from build123d import *

# Parameters (mm, degrees)
SKETCH3_W          = 8.5
SKETCH3_H          = 1
CUT_EXTRUDE1_DEPTH = 12.4
CUT_EXTRUDE2_DEPTH = 12.4


with BuildPart() as part:
    # Sketch1 → Revolve1 (revolve)
    with BuildSketch(Plane(origin=(0, 0, 0), x_dir=(0, 0, -1), z_dir=(1, 0, 0)), mode=Mode.PRIVATE) as revolve1_sk:
        with BuildLine():
            Line((-12.4, 7), (-12.4, 3.675))
            Line((-12.4, 3.675), (-11.9, 3.175))
            Line((-11.9, 3.175), (-0.5, 3.175))
            Line((-0.5, 3.175), (0, 3.675))
            Line((0, 3.675), (0, 8))
            Line((0, 8), (-0.5, 8.5))
            Line((-0.5, 8.5), (-2.2, 8.5))
            Line((-2.2, 8.5), (-2.2, 8.3))
            Line((-2.2, 8.3), (-4.4, 8.3))
            Line((-4.4, 8.3), (-4.4, 8.5))
            Line((-4.4, 8.5), (-7, 8.5))
            Line((-7, 8.5), (-7, 8.1))
            ThreePointArc((-7, 8.1), (-7.175735931, 7.675735931), (-7.6, 7.5))
            Line((-7.6, 7.5), (-11.9, 7.5))
            Line((-11.9, 7.5), (-12.4, 7))
        make_face()
    revolve(revolve1_sk.sketch.rotate(Axis((0, 0, 0), (0, 0, 1)), 270), axis=Axis((0, 0, 0), (0, 0, 1)))

    # Sketch2 → Cut-Revolve1 (revolve, cut)
    with BuildSketch(Plane.XY.offset(3), mode=Mode.PRIVATE) as cut_revolve1_sk:
        Polygon((-6, 8.5), (-3.5, 8.5), (-3.5, 2.3), (-4.9935, 2.3), (-4.9935, -8.5), (-6, -8.5), align=None)
    revolve(cut_revolve1_sk.sketch.rotate(Axis((-6, -8.5, 3), (0, 1, 0)), 270), axis=Axis((-6, -8.5, 3), (0, 1, 0)), mode=Mode.SUBTRACT)

    # Sketch3 → Cut-Extrude1 (cut)
    with BuildSketch(Plane.XY):
        with Locations((-4.25, 0)):
            Rectangle(SKETCH3_W, SKETCH3_H)
    extrude(amount=CUT_EXTRUDE1_DEPTH, mode=Mode.SUBTRACT)

    # Sketch4 → Cut-Extrude2 (cut)
    with BuildSketch(Plane.XY.offset(7)):
        with BuildLine():
            ThreePointArc((-1.710892857, 4.431178808), (-13.9, 0), (-1.710892857, -4.431178808))
            ThreePointArc((-1.710892857, -4.431178808), (0, -4.75), (1.710892857, -4.431178808))
            ThreePointArc((1.710892857, -4.431178808), (13.9, 0), (1.710892857, 4.431178808))
            ThreePointArc((1.710892857, 4.431178808), (0, 4.75), (-1.710892857, 4.431178808))
        make_face()
    extrude(amount=CUT_EXTRUDE2_DEPTH, mode=Mode.SUBTRACT)


solid = part.part
Design review of the part built by this model. Coordinates are the model's own, in mm. A direction names the side the tool comes from. Coordinates: 2 decimals unless noted, no trailing zeros. Loops run counter-clockwise (first coordinate to the right, second up) from the corner with the lowest first, then second, coordinate; pieces in that order, holes last.
Item 1: Draft analysis for pull direction Z (two halves, no side actions). For faces 1 (the flat face through (-7, 2.3, 2)), 2 (the cylindrical face through (0.02, 4.75, 9.66)), 3 (the flat face through (1.9, -3.4, 0)), state which applies: pulls with the +Z half, pulls with the -Z half, needs draft (parallel to the pull), parting line crosses it, or undercut.
Completed:
face 1: undercut
face 2: needs draft
face 3: pulls with the -Z half
Item 2: Clearance check with flat-ended pins moving along their axes: pin 1 (1.5 mm diameter, centred on x = -8, y = -4, fed in from +Z); pin 2 (4 mm diameter, centred on x = -0.5, z = 10.5, fed in from -Y); pin 3 (2.5 mm diameter, centred on x = -6, z = 3, fed in from +Y); pin 4 (1.6 mm diameter, centred on x = -6, z = 3, fed in from +Y). State where each tip first meets the part, or that it passes through.
Completed:
pin 1: stops at z = 7
pin 2: stops at y = -7.5
pin 3: stops at y = 2.3
pin 4: passes through
Item 3: Add section D-D (z = 3). Give the number of separate pieces and of enclosed holes in the cut face, and give its area (3 significant figures).
Completed:
separate pieces: 3
enclosed holes: 0
area: 150 mm2
Item 4: Wall thickness on L1, parallel to Y at x = 0, z = 3.25 (3 decimals); L2, parallel to Z at x = -6, y = -2; L3, parallel to X at y = 2, z = 3.25: over which ranges is each line inside the solid? List them lowest first.
Completed:
L1: y = -8.3 to -3.175, 3.175 to 8.3
L2: z = 0 to 1.99, 4.01 to 7
L3: x = -8.06 to -6.97, -5.03 to -2.47, 2.47 to 8.06
Item 5: For faces 4 (the cylindrical face through (-0.1, -7.5, 9.8)), 5 (the cylindrical face through (8.297, 0.224, 3.315)), 6 (the cylindrical face through (2.786, 5.464, 9.662)), 7 (the cylindrical face through (-2.786, -5.464, 9.662)), list the 3-axis set-ups (+Z, -Z, +X, -X, +Y, -Y) from which the entire face can be reached by the end or side of a thin tool; tool diameter is ignored.
Completed:
face 4: +Z, -Y
face 5: none
face 6: +Z, +X
face 7: +Z, -X
Item 6: Add section C-C (y = 0). Write out the cut boundary in (x, z) (3 decimals), and give its area (3 significant figures).
Completed:
outline: (3.175, 0.5) - (3.675, 0) - (8, 0) - (8.5, 0.5) - (8.5, 2.2) - (8.3, 2.2) - (8.3, 4.4) - (8.5, 4.4) - (8.5, 7) - (3.175, 7) - close
area: 36.6 mm2
Item 7: Add section A-A (z = 10.25). Write out the cut boundary in (x, y).
Completed:
outline: (-4.12, -6.27) arc R7.5 ccw to (4.12, -6.27) arc R6.9 cw to (1.71, -4.43) arc R4.75 cw to (-1.71, -4.43) arc R6.9 cw to start; (-4.12, 6.27) arc R6.9 cw to (-1.71, 4.43) arc R4.75 cw to (1.71, 4.43) arc R6.9 cw to (4.12, 6.27) arc R7.5 ccw to start
